Build history of the part. All positions in model axes, mm. A direction names the side the tool comes from. Give positions to 0.01 mm unless a question says otherwise; leave off trailing zeros. Order: outer loops, then holes, each group sorted by start corner. A loop starts at its lowest first (then second) coordinate and runs counter-clockwise, first axis right, second up. Notation, with made-up numbers: (-27.75, 86.5) - (-6.75, 86.5) arc R36 cw to (-6.75, 125.5) - close; hole circle Ø8 at (42.25, 76.25). An arc over 180 degrees is marked (long way). Use a Markdown table: item, result. Add a question column.
(1) Wall check: line 1 (X direction, y = 0, z = -6.5); line 2 (Y direction, x = 0, z = 0.75). Give the ranges that are in metal, low to high.
(2) Slice it at D-D (z = -1.5). Write the cut outline in (x, y) (3 decimals), then the cut area to 3 significant figures.
(3) Slice it at B-B (y = 0). Write the cut outline in (x, z) (3 decimals), then the cut area to 3 significant figures.
(4) Flat gauge pin, fed straight in: pin 1 (1.5 mm diameter, centred on x = 0, z = -6, fed in from +Y). Where does the tip first touch, or does it go through?
(5) Slice it at C-C (x = 0). Write the cut outline in (y, z) (3 decimals), then the cut area to 3 significant figures.
(6) Which spindle directions (+Z, -Z, +X, -X, +Y, -Y) get a long thin tool onto all of the face, cutting with end or side? Do faces 1 (the face through (-0.8, -1.5, -4.826)), 2 (the face through (-1.588, -3.3, -4.1)), 3 (the face through (1.588, -3.3, -4.1)), 4 (the face through (-0.5, -2.23, 0.61)). Say none if no direction does.
from build123d import *

# Parameters (mm, degrees)
F0_R     = 2.286
F1_DEPTH = 1.5
F2_R     = 3.175
F2_R_2   = 2.286
F3_DEPTH = 4.826
F4_SIZE  = 0.254
F5_R     = 1.524
F6_DEPTH = 2.54
F7_W     = 3.175
F7_H     = 1.5
F8_DEPTH = 4.318
F9_R     = 0.508
F10_SIZE = 0.254
F11_R    = 0.254
F12_SIZE = 0.254


# Not quite as in the source:
# - a feature names something its author has since deleted; it is built from what else it names


with BuildPart() as f1:
    # F0 (on Top) → F1 (new body)
    with BuildSketch(Plane.XY):
        Circle(F0_R)
    extrude(amount=F1_DEPTH)

    # F2 (on face) → F3 (join)
    with BuildSketch(Plane(origin=(0, 0, 0), x_dir=(1, 0, 0), z_dir=(0, 0, -1))):
        Circle(F2_R)
        Circle(F2_R_2, mode=Mode.SUBTRACT)
        Circle(F2_R_2)
    extrude(amount=F3_DEPTH)

    # F4
    f4_edges = [f1.edges().sort_by_distance(p)[0] for p in [
        (-2.286, 0, 1.5),
    ]]
    chamfer(f4_edges, length=F4_SIZE)

    # F5 (on face) → F6 (join)
    with BuildSketch(Plane(origin=(0, 0, -4.826), x_dir=(1, 0, 0), z_dir=(0, 0, -1))):
        Circle(F5_R)
    extrude(amount=F6_DEPTH)

    # F7 (on Front) → F8 (join)
    with BuildSketch(Plane.XZ):
        with Locations((0, -4.076)):
            Rectangle(F7_W, F7_H)
    extrude(amount=F8_DEPTH)

    # F9
    f9_edges = [f1.edges().sort_by_distance(p)[0] for p in [
        (-1.5875, -4.318, -4.076),
        (1.5875, -4.318, -4.076),
    ]]
    fillet(f9_edges, radius=F9_R)

    # F10
    f10_edges = [f1.edges().sort_by_distance(p)[0] for p in [
        (-1.524, 0, -7.366),
    ]]
    chamfer(f10_edges, length=F10_SIZE)

    # F11
    f11_edges = [f1.edges().sort_by_distance(p)[0] for p in [
        (0, -3.175, -3.326),
        (1.5875, -2.749631, -4.076),
        (-1.5875, -2.749631, -4.076),
    ]]
    fillet(f11_edges, radius=F11_R)

    # F12
    f12_edges = [f1.edges().sort_by_distance(p)[0] for p in [
        (-3.175, 0, 0),
    ]]
    chamfer(f12_edges, length=F12_SIZE)


solid = f1.part
Solution:
| question | item | result |
|---|---|---|
| 1 | line 1 | -1.52 to 1.52 |
| 1 | line 2 | -2.29 to 2.29 |
| 2 | outline | circle Ø6.35 at (0, 0) |
| 2 | area | 31.7 mm2 |
| 3 | outline | (-3.175, -4.826) - (-1.524, -4.826) - (-1.524, -7.112) - (-1.27, -7.366) - (1.27, -7.366) - (1.524, -7.112) - (1.524, -4.826) - (3.175, -4.826) - (3.175, -0.254) - (2.921, 0) - (2.286, 0) - (2.286, 1.246) - (2.032, 1.5) - (-2.032, 1.5) - (-2.286, 1.246) - (-2.286, 0) - (-2.921, 0) - (-3.175, -0.254) - close |
| 3 | area | 45.1 mm2 |
| 4 | pin 1 | y = 1.52 |
| 5 | outline | (-4.318, -4.826) - (-1.524, -4.826) - (-1.524, -7.112) - (-1.27, -7.366) - (1.27, -7.366) - (1.524, -7.112) - (1.524, -4.826) - (3.175, -4.826) - (3.175, -0.254) - (2.921, 0) - (2.286, 0) - (2.286, 1.246) - (2.032, 1.5) - (-2.032, 1.5) - (-2.286, 1.246) - (-2.286, 0) - (-2.921, 0) - (-3.175, -0.254) - (-3.175, -3.072) arc R0.254 cw to (-3.429, -3.326) - (-4.318, -3.326) - close |
| 5 | area | 46.8 mm2 |
| 6 | face 1 | -Z |
| 6 | face 2 | +Z, -Z, -X, -Y |
| 6 | face 3 | +Z, -Z, +X, -Y |
| 6 | face 4 | +Z |
